from build123d import *

# Parameters (mm, degrees)
BOSS_EXTRUDE1_DEPTH = 3
FILLET1_R           = 200
FILLET2_R           = 10
SKETCH2_R           = 30
CUT_EXTRUDE1_DEPTH  = 429.345808882
SKETCH3_W           = 66
SKETCH3_H           = 15
SKETCH3_R           = 1.6
BOSS_EXTRUDE2_DEPTH = 3
FILLET3_R           = 5
SKETCH4_R           = 1.6
CUT_EXTRUDE2_DEPTH  = 435.224748243
SKETCH5_R           = 1.6
CUT_EXTRUDE3_DEPTH  = 435.224748243
SKETCH7_R           = 1.6
CUT_EXTRUDE4_DEPTH  = 435.224748243
SKETCH8_R           = 1.6
CUT_EXTRUDE5_DEPTH  = 10


with BuildPart() as part:
    # Sketch1 → Boss-Extrude1 (new body)
    with BuildSketch(Plane(origin=(0, 0, 0), x_dir=(1, 0, 0), z_dir=(0, 1, 0))):
        Polygon((0, 0), (170, 0), (170, 300), (225, 300), (225, 367.51288694), (85, 330), (-55, 367.51288694), (-55, 300), (0, 300), align=None)
    extrude(amount=BOSS_EXTRUDE1_DEPTH)

    # Fillet1
    fillet1_edges = [part.edges().sort_by_distance(p)[0] for p in [
        (85, 1.5, -330),
    ]]
    fillet(fillet1_edges, radius=FILLET1_R)

    # Fillet2
    fillet2_edges = [part.edges().sort_by_distance(p)[0] for p in [
        (0, 1.5, -300),
        (-55, 1.5, -300),
        (-55, 1.5, -367.51288694),
        (225, 1.5, -367.51288694),
        (225, 1.5, -300),
        (170, 1.5, -300),
        (170, 1.5, 0),
        (0, 1.5, 0),
    ]]
    fillet(fillet2_edges, radius=FILLET2_R)

    # Sketch2 → Cut-Extrude1 (cut, through all)
    with BuildSketch(Plane(origin=(0, 3, 0), x_dir=(1, 0, 0), z_dir=(0, 1, 0))):
        with Locations(Location((85, 80, 0), (0, 0, 270))):
            Circle(SKETCH2_R)
    extrude(amount=-CUT_EXTRUDE1_DEPTH, mode=Mode.SUBTRACT)

    # Sketch3 → Boss-Extrude2 (add)
    # profile 1 of 2: a face of its own
    with BuildSketch(Plane(origin=(0, 3, 0), x_dir=(1, 0, 0), z_dir=(0, 1, 0))):
        with Locations((-33, 52.5)):
            Rectangle(SKETCH3_W, SKETCH3_H)
        with Locations(Location((-21, 52.5, 0), (0, 0, 270))):
            Circle(SKETCH3_R, mode=Mode.SUBTRACT)
        with Locations(Location((-45, 52.5, 0), (0, 0, 270))):
            Circle(SKETCH3_R, mode=Mode.SUBTRACT)
    # profile 2 of 2: a face of its own
    with BuildSketch(Plane(origin=(0, 3, 0), x_dir=(1, 0, 0), z_dir=(0, 1, 0))):
        with Locations((203, 52.5)):
            Rectangle(SKETCH3_W, SKETCH3_H)
        with Locations(Location((191, 52.5, 0), (0, 0, 90))):
            Circle(SKETCH3_R, mode=Mode.SUBTRACT)
        with Locations(Location((215, 52.5, 0), (0, 0, 90))):
            Circle(SKETCH3_R, mode=Mode.SUBTRACT)
    extrude(amount=-BOSS_EXTRUDE2_DEPTH)

    # Fillet3
    fillet3_edges = [part.edges().sort_by_distance(p)[0] for p in [
        (0, 1.5, -60),
        (0, 1.5, -45),
        (-66, 1.5, -45),
        (-66, 1.5, -60),
        (170, 1.5, -45),
        (170, 1.5, -60),
        (236, 1.5, -60),
        (236, 1.5, -45),
    ]]
    fillet(fillet3_edges, radius=FILLET3_R)

    # Sketch4 → Cut-Extrude2 (cut, through all)
    with BuildSketch(Plane.XZ):
        with Locations(Location((162.5, -7.5, 0), (0, 0, 270))):
            Circle(SKETCH4_R)
        with Locations(Location((162.5, -52.5, 0), (0, 0, 270))):
            Circle(SKETCH4_R)
        with Locations(Location((100, -7.5, 0), (0, 0, 270))):
            Circle(SKETCH4_R)
        with Locations(Location((70, -7.5, 0), (0, 0, 270))):
            Circle(SKETCH4_R)
        with Locations(Location((162.5, -97.5, 0), (0, 0, 270))):
            Circle(SKETCH4_R)
        with Locations(Location((162.5, -222.3, 0), (0, 0, 270))):
            Circle(SKETCH4_R)
        with Locations(Location((162.5, -267.3, 0), (0, 0, 270))):
            Circle(SKETCH4_R)
        with Locations(Location((162.5, -312, 0), (0, 0, 270))):
            Circle(SKETCH4_R)
        with Locations(Location((162.5, -342.75495241, 0), (0, 0, 270))):
            Circle(SKETCH4_R)
        with Locations(Location((109.337835254, -328.510193298, 0), (0, 0, 270))):
            Circle(SKETCH4_R)
        with Locations(Location((60.662164746, -328.510193298, 0), (0, 0, 270))):
            Circle(SKETCH4_R)
        with Locations(Location((7.5, -342.75495241, 0), (0, 0, 270))):
            Circle(SKETCH4_R)
        with Locations(Location((7.5, -312, 0), (0, 0, 270))):
            Circle(SKETCH4_R)
        with Locations(Location((7.5, -267.3, 0), (0, 0, 270))):
            Circle(SKETCH4_R)
        with Locations(Location((7.5, -222.3, 0), (0, 0, 270))):
            Circle(SKETCH4_R)
        with Locations(Location((7.5, -97.5, 0), (0, 0, 270))):
            Circle(SKETCH4_R)
        with Locations(Location((7.5, -52.5, 0), (0, 0, 270))):
            Circle(SKETCH4_R)
        with Locations(Location((7.5, -7.5, 0), (0, 0, 270))):
            Circle(SKETCH4_R)
        with Locations(Location((70, -267.5, 0), (0, 0, 270))):
            Circle(SKETCH4_R)
        with Locations(Location((100, -267.5, 0), (0, 0, 270))):
            Circle(SKETCH4_R)
    extrude(amount=-CUT_EXTRUDE2_DEPTH, mode=Mode.SUBTRACT)

    # Sketch5 → Cut-Extrude3 (cut, through all)
    with BuildSketch(Plane(origin=(0, 3, 0), x_dir=(1, 0, 0), z_dir=(0, 1, 0))):
        with Locations(Location((-40.836994935, 355.953349818, 0), (0, 0, 270))):
            Circle(SKETCH5_R)
        with Locations(Location((-11.859220146, 348.188778465, 0), (0, 0, 270))):
            Circle(SKETCH5_R)
        with Locations(Location((182.234220146, 348.289259412, 0), (0, 0, 270))):
            Circle(SKETCH5_R)
        with Locations(Location((211.211994935, 356.053830765, 0), (0, 0, 270))):
            Circle(SKETCH5_R)
    extrude(amount=-CUT_EXTRUDE3_DEPTH, mode=Mode.SUBTRACT)

    # Sketch7 → Cut-Extrude4 (cut, through all)
    with BuildSketch(Plane(origin=(0, 3, 0), x_dir=(1, 0, 0), z_dir=(0, 1, 0))):
        with Locations(Location((-45, 327.5, 0), (0, 0, 270))):
            Circle(SKETCH7_R)
        with Locations(Location((-45, 307.5, 0), (0, 0, 270))):
            Circle(SKETCH7_R)
        with Locations(Location((-15, 327.5, 0), (0, 0, 270))):
            Circle(SKETCH7_R)
        with Locations(Location((-15, 307.5, 0), (0, 0, 270))):
            Circle(SKETCH7_R)
        with Locations(Location((185, 327.5, 0), (0, 0, 90))):
            Circle(SKETCH7_R)
        with Locations(Location((185, 307.5, 0), (0, 0, 90))):
            Circle(SKETCH7_R)
        with Locations(Location((215, 307.5, 0), (0, 0, 90))):
            Circle(SKETCH7_R)
        with Locations(Location((215, 327.5, 0), (0, 0, 90))):
            Circle(SKETCH7_R)
    extrude(amount=-CUT_EXTRUDE4_DEPTH, mode=Mode.SUBTRACT)

    # Sketch8 → Cut-Extrude5 (cut)
    with BuildSketch(Plane(origin=(0, 3, 0), x_dir=(1, 0, 0), z_dir=(0, 1, 0))):
        with Locations(Location((85, 133, 0), (0, 0, 270))):
            Circle(SKETCH8_R)
        with Locations(Location((122.476659403, 117.476659403, 0), (0, 0, 270))):
            Circle(SKETCH8_R)
        with Locations(Location((138, 80, 0), (0, 0, 270))):
            Circle(SKETCH8_R)
        with Locations(Location((122.476659403, 42.523340597, 0), (0, 0, 270))):
            Circle(SKETCH8_R)
        with Locations(Location((85, 27, 0), (0, 0, 270))):
            Circle(SKETCH8_R)
        with Locations(Location((47.523340597, 42.523340597, 0), (0, 0, 270))):
            Circle(SKETCH8_R)
        with Locations(Location((32, 80, 0), (0, 0, 270))):
            Circle(SKETCH8_R)
        with Locations(Location((47.523340597, 117.476659403, 0), (0, 0, 270))):
            Circle(SKETCH8_R)
    extrude(amount=-CUT_EXTRUDE5_DEPTH, mode=Mode.SUBTRACT)


solid = part.part
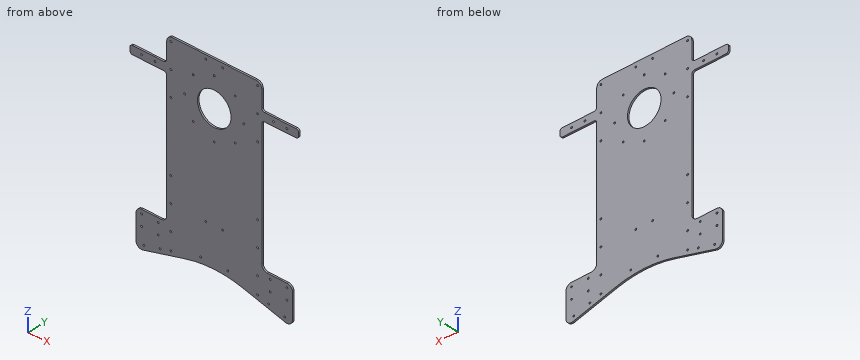
Could you check a few things on this model? Use its own coordinates, in mm. Coordinates: 2 decimals unless noted, no trailing zeros. Write each loop counter-clockwise with the first axis right and the second up, starting at its lowest first coordinate (ties: lowest second). Pieces come first, ordered by that corner, then holes. Notation, with made-up numbers: (54.25, 33) - (93.25, 33) arc R5 ccw to (93.25, 40) - close; hole circle Ø11 at (18, -25). An arc over 180 degrees is marked (long way). Put each result on its own line as item: value. Start each with the question number.
Q1. Please list where these lines run through material, in increasing order: L1, parallel to X at y = 1.8, z = -307.5; L2, parallel to X at y = 1.2, z = -239; L3, parallel to Z at x = 11, y = 1.8.
Q2. I want a section at A-A on z = -86.5. Write out the boundary of the cut face in (x, y).
Q3. I want a section at C-C on x = 17.5. Write out the boundary of the cut face in (y, z).
Q4. I'm going to push flat-ended pins straight in: P1, Ø3.5, axis at x = 215, z = -327.5, coming from the -Y side; P2, Ø0.9, axis at y = 2, z = -121.5, coming from the +X side; P3, Ø1, axis at x = 53, y = 0.5, coming from the -Z side; P4, Ø1.9, axis at x = 122.48, z = -117.48, coming from the -Y side. Where does each tip first touch, or does it pass through?
Q5. I want a section at B-B on y = 2.15. Count the separate pieces of the cut face and the enclosed holes in it, plus the area to 3 significant figures.
Checks:
1. L1: -54.68 to -46.6, -43.4 to -16.6, -13.4 to 183.4, 186.6 to 213.4, 216.6 to 224.68
1. L2: 0 to 170
1. L3: -349.83 to 0
2. outline: (0, 0) - (55.71, 0) - (55.71, 3) - (0, 3) - close; (114.29, 0) - (170, 0) - (170, 3) - (114.29, 3) - close
3. outline: (0, -348.09) - (3, -348.09) - (3, 0) - (0, 0) - close
4. P1: y = 0
4. P2: x = 170
4. P3: z = -339.71
4. P4: through
5. separate pieces: 1
5. enclosed holes: 45
5. area: 63,600 mm²
